Design review of the part shown in the three views and the two pictorial views. Dimensions are in mm from the part's minimum x, y and z. A direction names the side the tool comes from. Round coordinates to 2 decimals unless told otherwise and drop trailing zeros. Write each loop counter-clockwise with the first axis right and the second up, starting at its lowest first coordinate (ties: lowest second). Pieces come first, ordered by that corner, then holes. Notation, with made-up numbers: (62.25, -31.75) -> (80.25, -31.75) arc R24 cw to (80.25, -1.75) -> close; hole circle Ø3 at (-12.75, 62.5). An arc over 180 degrees is marked (long way). Return JSON: item names as keys, results as strings. Group by question number.
1. For line 1 along Y through (x, z) = (51.25, 27.6); line 2 along X through (y, z) = (15.5, 28); line 3 along Z through (x, y) = (24, 6.75), list the stretches that pass through material, from the lowest coordinate up. Write a range as from..to.
2. Take a section at D-D, the plane z = 9.5. Write out the cut boundary in (x, y), then the cut area to 3 significant figures.
3. Take a section at B-B, the plane y = 4.75. Write out the cut boundary in (x, z), then the cut area to 3 significant figures.
4. Take a section at A-A, the plane x = 2.75. Write out the cut boundary in (y, z).
5. Tool access review of the marked faces 1, 2, 3 and 4: name each direction out of +Z, -Z, +X, -X, +Y, -Y from which nothing blocks a thin tool from reaching the whole face with its end or side.
6. Clearance check with flat-ended pins moving along their axes: P1, Ø4, axis at y = 8, z = 20.5, coming from the -X side; P2, Ø1.6, axis at x = 35, z = 36, coming from the -Y side; P3, Ø6, axis at x = 51.25, y = 14.25, coming from the +Z side. State where each tip first meets the part, or that it passes through.
7. Take a section at C-C, the plane x = 34. Write out the cut boundary in (y, z).
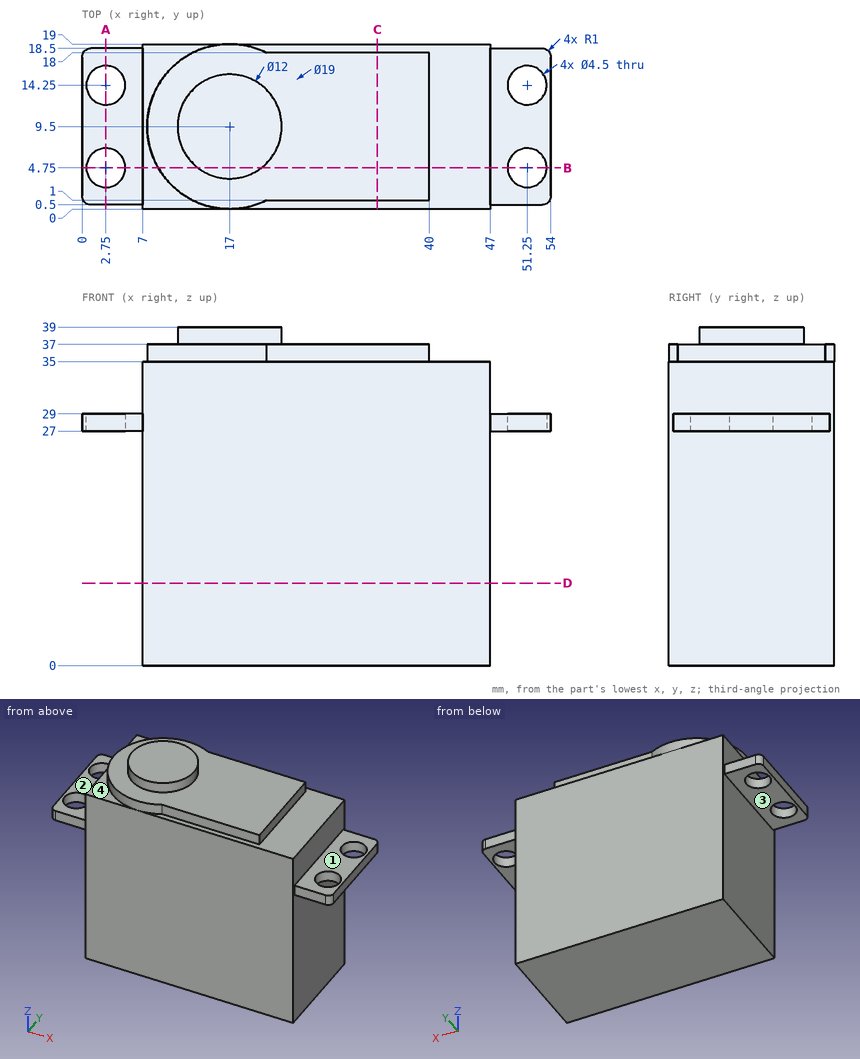
Output:
{
 "1": {"line 1": "y = 0.5..2.5, 7..12, 16.5..18.5", "line 2": "x = 0..0.88, 4.62..49.38, 53.12..54", "line 3": "z = 0..37"},
 "2": {"outline": "(7, 0) -> (47, 0) -> (47, 19) -> (7, 19) -> close", "area": "760 mm^2"},
 "3": {"outline": "(0, 27) -> (0.5, 27) -> (0.5, 29) -> (0, 29) -> close; (5, 27) -> (7, 27) -> (7, 0) -> (47, 0) -> (47, 27) -> (49, 27) -> (49, 29) -> (47, 29) -> (47, 35) -> (40, 35) -> (40, 37) -> (20.67, 37) -> (20.67, 39) -> (13.33, 39) -> (13.33, 37) -> (8.77, 37) -> (8.77, 35) -> (7, 35) -> (7, 29) -> (5, 29) -> close; (53.5, 27) -> (54, 27) -> (54, 29) -> (53.5, 29) -> close", "area": "1,490 mm^2"},
 "4": {"outline": "(0.5, 27) -> (2.5, 27) -> (2.5, 29) -> (0.5, 29) -> close; (7, 27) -> (12, 27) -> (12, 29) -> (7, 29) -> close; (16.5, 27) -> (18.5, 27) -> (18.5, 29) -> (16.5, 29) -> close"},
 "5": {"face 1": "+Z, +X, +Y, -Y", "face 2": "+Z, -X, +Y, -Y", "face 3": "-Z, -X, +Y, -Y", "face 4": "+Z, -X"},
 "6": {"P1": "stops at x = 7", "P2": "stops at y = 1", "P3": "stops at z = 29"},
 "7": {"outline": "(0, 0) -> (19, 0) -> (19, 35) -> (18, 35) -> (18, 37) -> (1, 37) -> (1, 35) -> (0, 35) -> close"}
}
